Part model, mm, in its own coordinate system. Round coordinates to 2 decimals unless told otherwise and drop trailing zeros. Write each loop counter-clockwise with the first axis right and the second up, starting at its lowest first coordinate (ties: lowest second). Pieces come first, ordered by that corner, then holes. Notation, with made-up numbers: (-11, 63) -> (41, 63) arc R24 cw to (41, 91) -> close; hole circle Ø11 at (-10.75, 5). An arc over 180 degrees is marked (long way). Use CSV: the item, a comma, the result in double quotes. Start each with the question number.
(1) Drop flat-ended pins along their axis: pin 1 (2.5 mm diameter, centred on x = -0.5, z = -1, fed in from -Y); pin 2 (2 mm diameter, centred on x = 3, y = 491, fed in from -Z); pin 3 (4 mm diameter, centred on x = 0, z = 0, fed in from +Y) (3 decimals). Give the stop position or say it passes through.
(2) Saw through at B-B (y = 429). Give the cut face in (x, z), plus the area to 3 significant figures.
(3) Probe line 1 (Z direction, x = 0, y = 18.5); line 2 (X direction, y = 709.5, z = 0); line 3 (Z direction, x = -5, y = 302). List the from-to ranges inside material, lowest first. Write a range as [from, to].
(4) Saw through at A-A (z = 0). Give the cut face in (x, y) (3 decimals).
Autodesk Inventor part; units mm, degrees
ref_plane "YZ Plane" through (0, 0, 0) normal (1, 0, 0) x (0, 1, 0)
ref_plane "XZ Plane" through (0, 0, 0) normal (0, 1, 0) x (-1, 0, 0)
ref_plane "XY Plane" through (0, 0, 0) normal (0, 0, 1) x (1, 0, 0)
sketch "Sketch1" plane through (0, 0, 0) normal (0, 1, 0) x (-1, 0, 0)
  line L0 (6.35, -3.6662) -> (0, -7.3323)
  line L1 (0, -7.3323) -> (-6.35, -3.6662)
  line L2 (-6.35, -3.6662) -> (-6.35, 3.6662)
  line L3 (-6.35, 3.6662) -> (0, 7.3323)
  line L4 (0, 7.3323) -> (6.35, 3.6662)
  line L5 (6.35, 3.6662) -> (6.35, -3.6662)
  point P0 (0, 0)
  point P1 (0, 0)
  point P2 (0, 0)
  dimension "d0" = 12.7
extrude "Extrusion1" add sketch "Sketch1" along normal blind 714.375
sketch "Sketch2" plane through (0, 0, 0) normal (0, -1, 0) x (1, 0, 0)
  point P0 (0, 0)
  point P1 (0, 0)
hole "Hole1" at (0, 0, 0) direction (0, 1, 0) diameter 4.9784 depth 25.4
sketch "Sketch3" plane through (0, 714.375, 0) normal (0, 1, 0) x (1, 0, 0)
  point P0 (0, 0)
  point P1 (0, 0)
hole "Hole2" at (0, 714.375, 0) direction (0, -1, 0) diameter 4.9784 depth 25.4
properties part number "Intake HexShaft 2" material "Aluminum 7075"
Answers:
1,pin 1,"stops at y = 25.4"
1,pin 2,"stops at z = -6.18"
1,pin 3,"stops at y = 688.975"
2,outline,"(-6.35, -3.67) -> (0, -7.33) -> (6.35, -3.67) -> (6.35, 3.67) -> (0, 7.33) -> (-6.35, 3.67) -> close"
2,area,"140 mm²"
3,line 1,"z = [-7.33, -2.49], [2.49, 7.33]"
3,line 2,"x = [-6.35, -2.49], [2.49, 6.35]"
3,line 3,"z = [-4.45, 4.45]"
4,outline,"(-6.35, 0) -> (-2.489, 0) -> (-2.489, 25.4) -> (2.489, 25.4) -> (2.489, 0) -> (6.35, 0) -> (6.35, 714.375) -> (2.489, 714.375) -> (2.489, 688.975) -> (-2.489, 688.975) -> (-2.489, 714.375) -> (-6.35, 714.375) -> close"
